Check sheet for the modelled part. Datum: model origin and axes. Units: mm. A direction names the side the tool comes from. Round coordinates to 2 decimals unless told otherwise and drop trailing zeros. Order: outer loops, then holes, each group sorted by start corner. A loop starts at its lowest first (then second) coordinate and runs counter-clockwise, first axis right, second up. Notation, with made-up numbers: (-14, 7.5) -> (25, 7.5) arc R6 cw to (25, 17.5) -> close; hole circle Ø1 at (-38, -27.75). An arc over 180 degrees is marked (long way). Use CSV: the item, a comma, the result in double quotes.
```python
from build123d import *

# Parameters (mm, degrees)
SKETCH_1_R          = 1
SKETCH_1_R_2        = 1.55
SKETCH_1_R_3        = 6
EXTRUDE_1_DEPTH     = 20
CUT_EXTRUDE_1_DEPTH = 33.5
CUT_EXTRUDE_2_DEPTH = 21


with BuildPart() as part:
    # 草图1 → 凸台-拉伸1 (new body)
    with BuildSketch(Plane.XY):
        Polygon((10, 0), (10, 12.5), (0, 12.5), (-10, 12.5), (-10, -24), (10, -24), align=None)
        Circle(SKETCH_1_R, mode=Mode.SUBTRACT)
        with Locations((0, 4)):
            Circle(SKETCH_1_R_2, mode=Mode.SUBTRACT)
        with Locations((4, 0)):
            Circle(SKETCH_1_R_2, mode=Mode.SUBTRACT)
        with Locations((0, -4)):
            Circle(SKETCH_1_R_2, mode=Mode.SUBTRACT)
        with Locations((-4, 0)):
            Circle(SKETCH_1_R_2, mode=Mode.SUBTRACT)
        with Locations((0, -11.97364961)):
            Circle(SKETCH_1_R_3, mode=Mode.SUBTRACT)
    extrude(amount=EXTRUDE_1_DEPTH)

    # 草图2 → 切除-拉伸1 (cut)
    with BuildSketch(Plane(origin=(0, 12.5, 0), x_dir=(1, 0, 0), z_dir=(0, 1, 0))):
        Polygon((-7.7, -10.2), (-7.7, -2.5), (0, -2.5), (7.7, -2.5), (7.7, -17.9), (0, -17.9), (-7.7, -17.9), align=None)
    extrude(amount=-CUT_EXTRUDE_1_DEPTH, mode=Mode.SUBTRACT)

    # 草图3 → 切除-拉伸2 (cut, through all)
    with BuildSketch(Plane.ZY.offset(10)):
        with BuildLine():
            ThreePointArc((16, -5.75), (14.242640687, -1.507359313), (10, 0.25))
            Line((10, 0.25), (10, -11.75))
            ThreePointArc((10, -11.75), (14.242640687, -9.992640687), (16, -5.75))
        make_face()
        with BuildLine():
            Line((10, -11.75), (10, 0.25))
            ThreePointArc((10, 0.25), (4, -5.75), (10, -11.75))
        make_face()
        with BuildLine():
            ThreePointArc((15, 6.688097559), (13.535533906, 10.223631465), (10, 11.688097559))
            Line((10, 11.688097559), (10, 1.688097559))
            ThreePointArc((10, 1.688097559), (13.535533906, 3.152563653), (15, 6.688097559))
        make_face()
        with BuildLine():
            Line((10, 1.688097559), (10, 11.688097559))
            ThreePointArc((10, 11.688097559), (5, 6.688097559), (10, 1.688097559))
        make_face()
        with BuildLine():
            ThreePointArc((14, -15.973088327), (12.828427125, -13.144661202), (10, -11.973088327))
            Line((10, -11.973088327), (10, -19.973088327))
            ThreePointArc((10, -19.973088327), (12.828427125, -18.801515451), (14, -15.973088327))
        make_face()
        with BuildLine():
            Line((10, -19.973088327), (10, -11.973088327))
            ThreePointArc((10, -11.973088327), (6, -15.973088327), (10, -19.973088327))
        make_face()
    extrude(amount=-CUT_EXTRUDE_2_DEPTH, mode=Mode.SUBTRACT)


solid = part.part
```
Q1. Mould release check, pull along X, two halves, no side actions. Record for faces 1 (the face through (-10, -5, 3)), 2 (the face through (0, 12.5, 19)), 3 (the face through (7.7, 0, 7)): pulls with the +X half, pulls with the -X half, needs draft (parallel to the pull), parting line crosses it, or undercut.
Result sheet:
face 1,"pulls with the -X half"
face 2,"needs draft"
face 3,"undercut"
Q2. Sectioned sample at C-C, the plane z = 12.75. State how many separate pieces and enclosed holes the cut face has, then the cut area to 3 significant figures.
Result sheet:
separate pieces,"7"
enclosed holes,"0"
area,"99.9 mm^2"
Q3. Sectioned sample at B-B, the plane x = -4. Enter the section's corners in (y, z), then the cut area to 3 significant figures.
Result sheet:
outline,"(-24, 0) -> (-16.45, 0) -> (-16.45, 2.5) -> (-21, 2.5) -> (-21, 17.9) -> (-16.45, 17.9) -> (-16.45, 20) -> (-24, 20) -> close; (-7.5, 0) -> (-1.55, 0) -> (-1.55, 2.5) -> (-7.5, 2.5) -> close; (-7.5, 17.9) -> (-1.55, 17.9) -> (-1.55, 20) -> (-7.5, 20) -> close; (1.55, 0) -> (12.5, 0) -> (12.5, 2.5) -> (1.55, 2.5) -> close; (1.55, 17.9) -> (12.5, 17.9) -> (12.5, 20) -> (1.55, 20) -> close"
area,"159 mm^2"
Q4. Sectioned sample at D-D, the plane y = -2. Enter the section's corners in (x, z), then the cut area to 3 significant figures.
Result sheet:
outline,"(-10, 0) -> (10, 0) -> (10, 5.32) -> (7.7, 5.32) -> (7.7, 2.5) -> (-7.7, 2.5) -> (-7.7, 5.32) -> (-10, 5.32) -> close; (-10, 14.68) -> (-7.7, 14.68) -> (-7.7, 17.9) -> (7.7, 17.9) -> (7.7, 14.68) -> (10, 14.68) -> (10, 20) -> (-10, 20) -> close"
area,"120 mm^2"
Q5. Scan lines: L1, parallel to X at y = 0, z = 1.85; L2, parallel to Y at x = 0, z = 19.05; L3, parallel to X at y = -4, z = 1.9. Record each from-to range of solid material in increasing order.
Result sheet:
L1,"x = -10 to -5.55, -2.45 to -1, 1 to 2.45, 5.55 to 10"
L2,"y = -24 to -17.97, -5.97 to -5.55, -2.45 to -1, 1 to 2.45, 5.55 to 12.5"
L3,"x = -10 to -1.55, 1.55 to 10"
Q6. Go/stop test with a flat-tipped pin: pin 1 (7.5 mm diameter, centred on x = -3, z = 7, fed in from +Y). Record where the tip stops, or that it passes through.
Result sheet:
pin 1,"stops at y = -21"
Q7. Access from +Z, -Z, +X, -X, +Y, -Y to the whole of each face (thin tool, end or side, straight path). Record for faces 4 (the face through (-2, 0, 17.9)), 5 (the face through (-0.781, -6.025, 1.232)).
Result sheet:
face 4,"+Y"
face 5,"+Z, -Z"
Q8. Sectioned sample at A-A, the plane y = -7. Enter the section's corners in (x, z), then the cut area to 3 significant figures.
Result sheet:
outline,"(-10, 0) -> (-3.36, 0) -> (-3.36, 2.5) -> (-7.7, 2.5) -> (-7.7, 4.13) -> (-10, 4.13) -> close; (-10, 15.87) -> (-7.7, 15.87) -> (-7.7, 17.9) -> (-3.36, 17.9) -> (-3.36, 20) -> (-10, 20) -> close; (3.36, 0) -> (10, 0) -> (10, 4.13) -> (7.7, 4.13) -> (7.7, 2.5) -> (3.36, 2.5) -> close; (3.36, 17.9) -> (7.7, 17.9) -> (7.7, 15.87) -> (10, 15.87) -> (10, 20) -> (3.36, 20) -> close"
area,"78.0 mm^2"
